Design review of the part built by this model. Coordinates are the model's own, in mm. Face numbers are marked on the shaded views. A direction names the side the tool comes from. Give positions to 0.01 mm unless a question says otherwise; leave off trailing zeros. Order: outer loops, then holes, each group sorted by start corner. A loop starts at its lowest first (then second) coordinate and runs counter-clockwise, first axis right, second up.
```python
from build123d import *

# Parameters (mm, degrees)
SKETCH_1_R          = 1.1
EXTRUDE_1_DEPTH     = 4
SKETCH_2_R          = 4
CUT_EXTRUDE_1_DEPTH = 2
FILLET_1_R          = 5


with BuildPart() as part:
    # 草图1 → 凸台-拉伸1 (new, symmetric)
    with BuildSketch(Plane(origin=(0, 0, 0), x_dir=(0, 0, -1), z_dir=(1, 0, 0))):
        with BuildLine():
            Line((-12.5, 2.5), (12.5, 2.5))
            ThreePointArc((12.5, 2.5), (15, 0), (12.5, -2.5))
            Line((12.5, -2.5), (-12.5, -2.5))
            ThreePointArc((-12.5, -2.5), (-15, 0), (-12.5, 2.5))
        make_face()
        with Locations((12.5, 0)):
            Circle(SKETCH_1_R, mode=Mode.SUBTRACT)
        with Locations((-12.5, 0)):
            Circle(SKETCH_1_R, mode=Mode.SUBTRACT)
    extrude(amount=EXTRUDE_1_DEPTH, both=True)

    # 草图2 → 切除-拉伸1 (cut, symmetric)
    with BuildSketch(Plane(origin=(0, 0, 0), x_dir=(0, 0, -1), z_dir=(1, 0, 0))):
        with BuildLine():
            ThreePointArc((-9.377501001, 2.5), (-8.725745372, 1.324764885), (-8.5, 0))
            Line((-8.5, 0), (-5.520616019, 2.5))
            Line((-5.520616019, 2.5), (-9.377501001, 2.5))
        make_face()
        with BuildLine():
            Line((-5.520616019, -2.5), (-8.5, 0))
            ThreePointArc((-8.5, 0), (-8.725745372, -1.324764885), (-9.377501001, -2.5))
            Line((-9.377501001, -2.5), (-5.520616019, -2.5))
        make_face()
        with Locations((-12.5, 0)):
            Circle(SKETCH_2_R)
        with Locations((12.5, 0)):
            Circle(SKETCH_2_R)
        with BuildLine():
            Line((9.377501001, 2.5), (5.520616019, 2.5))
            Line((5.520616019, 2.5), (8.5, 0))
            ThreePointArc((8.5, 0), (8.725745372, 1.324764885), (9.377501001, 2.5))
        make_face()
        with BuildLine():
            ThreePointArc((9.377501001, -2.5), (8.725745372, -1.324764885), (8.5, 0))
            Line((8.5, 0), (5.520616019, -2.5))
            Line((5.520616019, -2.5), (9.377501001, -2.5))
        make_face()
    extrude(amount=CUT_EXTRUDE_1_DEPTH, both=True, mode=Mode.SUBTRACT)

    # 圆角1
    # the kernel refuses this fillet: 5 mm, written as the material it takes off along each edge
    with BuildSketch(Plane(origin=(2, 0, -8.5), x_dir=(0, -0.6427876096865346, 0.766044443118982), z_dir=(-1, 0, 0))) as fillet_1_piece_1:
        with BuildLine():
            CenterArc((5.885460651, 4.584253576), FILLET_1_R, 170, 76.469935568)
            Line((0.961421886, 5.452494464), (0, 0))
            Line((0, 0), (3.889309567, 0))
        make_face()
    extrude(amount=4, mode=Mode.SUBTRACT)
    with BuildSketch(Plane(origin=(-2, 0, 8.5), x_dir=(0, -0.6427876096865349, -0.7660444431189818), z_dir=(1, 0, 0))) as fillet_1_piece_2:
        with BuildLine():
            CenterArc((5.53660798, 5), FILLET_1_R, 193.530064432, 76.469935568)
            Line((0.675371519, 3.830222216), (0, 0))
            Line((0, 0), (5.53660798, 0))
        make_face()
    extrude(amount=4, mode=Mode.SUBTRACT)


solid = part.part
```
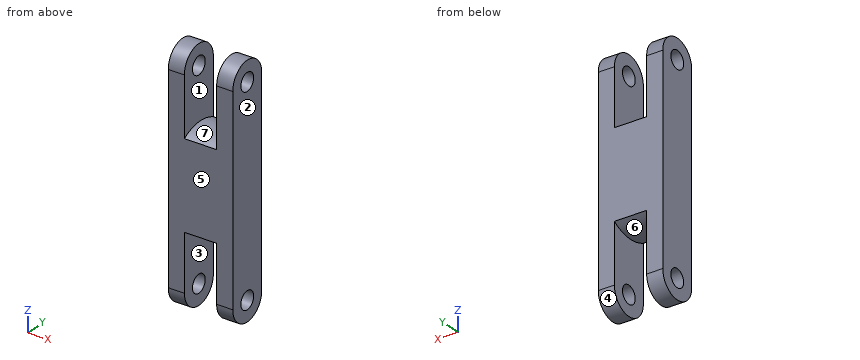
1. Take a section at D-D (y = 0). State the section outline as (x, z) points, then the cut area to 3 significant figures.
Recorded:
outline: (-4, -15) - (-2, -15) - (-2, -13.6) - (-4, -13.6) - close; (-4, -11.4) - (-2, -11.4) - (-2, -6.04) - (2, -6.04) - (2, -11.4) - (4, -11.4) - (4, 11.4) - (2, 11.4) - (2, 6.04) - (-2, 6.04) - (-2, 11.4) - (-4, 11.4) - close; (-4, 13.6) - (-2, 13.6) - (-2, 15) - (-4, 15) - close; (2, -15) - (4, -15) - (4, -13.6) - (2, -13.6) - close; (2, 13.6) - (4, 13.6) - (4, 15) - (2, 15) - close
area: 151 mm2
2. Take a section at C-C (z = -12). State the section outline as (x, y) points, then the cut area to 3 significant figures.
Recorded:
outline: (-4, -2.5) - (-2, -2.5) - (-2, -0.98) - (-4, -0.98) - close; (-4, 0.98) - (-2, 0.98) - (-2, 2.5) - (-4, 2.5) - close; (2, -2.5) - (4, -2.5) - (4, -0.98) - (2, -0.98) - close; (2, 0.98) - (4, 0.98) - (4, 2.5) - (2, 2.5) - close
area: 12.2 mm2
3. Take a section at B-B (x = -3). State the section outline as (y, z) points.
Recorded:
outline: (-2.5, -12.5) arc R2.5 ccw to (2.5, -12.5) - (2.5, 12.5) arc R2.5 ccw to (-2.5, 12.5) - close; hole circle Ø2.2 at (0, -12.5); hole circle Ø2.2 at (0, 12.5)
4. Machinability: for the marked faces 5, 6 and 7, which of the approach directions +Z, -Z, +X, -X, +Y, -Y give a long, thin tool a straight path to every point of the face, cutting with its end or side? Answer none if there is none.
Recorded:
face 5: +Z, -Z, +X, -X, -Y
face 6: -Z
face 7: +Z
5. Take a section at A-A (z = -9). State the section outline as (x, y) points, then the cut area to 3 significant figures.
Recorded:
outline: (-4, -2.5) - (-2, -2.5) - (-2, 2.5) - (-4, 2.5) - close; (2, -2.5) - (4, -2.5) - (4, 2.5) - (2, 2.5) - close
area: 20.0 mm2
6. For pin 1 (1.5 mm diameter, centred on x = 0.5, y = -1.5, fed in from +Z), flat-tipped, find the tip position at first contact; note if it passes through.
Recorded:
pin 1: stops at z = 5.94
7. Draft analysis for pull direction X (two halves, no side actions). For the marked faces 1, 2, 3 and 4, state which applies: pulls with the +X half, pulls with the -X half, needs draft (parallel to the pull), parting line crosses it, or undercut.
Recorded:
face 1: undercut
face 2: pulls with the +X half
face 3: undercut
face 4: needs draft
8. For line 1 along Z through (x, y) = (2.9, 0); line 2 along X through (y, z) = (0.95, -11.75); line 3 along Y through (x, z) = (-2.95, 12.5), list the stretches that pass through material, from the lowest coordinate up.
Recorded:
line 1: z = -15 to -13.6, -11.4 to 11.4, 13.6 to 15
line 2: x = -4 to -2, 2 to 4
line 3: y = -2.5 to -1.1, 1.1 to 2.5
